CAD build for the part. Positions are in the model's coordinates, mm. Face numbers are marked on the shaded views. A direction names the side the tool comes from. Coordinates: 2 decimals unless noted, no trailing zeros. Loops run counter-clockwise (first coordinate to the right, second up) from the corner with the lowest first, then second, coordinate; pieces in that order, holes last. Notation, with made-up numbers: (62, 0.5) -> (117, 0.5) arc R14 cw to (117, 7.5) -> close; hole circle Ø11 at (-31.5, -29). An arc over 180 degrees is marked (long way). Return JSON: item names as keys, results as strings. Group by question number.
(1) Flat gauge pins, fed straight in: pin 1 Ø4 at (x, y) = (-44, 44) entering from -Z; pin 2 Ø5 at (x, z) = (10, 10) entering from -Y; pin 3 Ø4.5 at (x, z) = (-9, 9) entering from -Y; pin 4 Ø16 at (x, z) = (63.5, 14.5) entering from -Y. Where does each tip first touch, or does it go through?
(2) Saw through at A-A on y = 12. Write the cut outline in (x, z), then the cut area to 3 significant figures.
(3) Saw through at D-D on x = 70. Write the cut outline in (y, z), then the cut area to 3 significant figures.
(4) Saw through at C-C on z = 24. Write the cut outline in (x, y).
(5) Tool access for the marked faces 1, 2, 3 and 4: list every direction of +Z, -Z, +X, -X, +Y, -Y with a clear straight run to the whole face (end or side of a thin tool).
(6) Probe L1, parallel to Z at x = 10, y = -51.2; L2, parallel to Y at x = 0, z = 23.5; L3, parallel to X at y = 22.5, z = 14. List the from-to ranges inside material, lowest first.
(7) Mould opens along Y. For the marked faces 5, 6 and 7 say: pulls with the +Y half, pulls with the -Y half, needs draft (parallel to the pull), parting line crosses it, or undercut.
(8) Saw through at B-B on x = -24. Write the cut outline in (y, z), then the cut area to 3 significant figures.
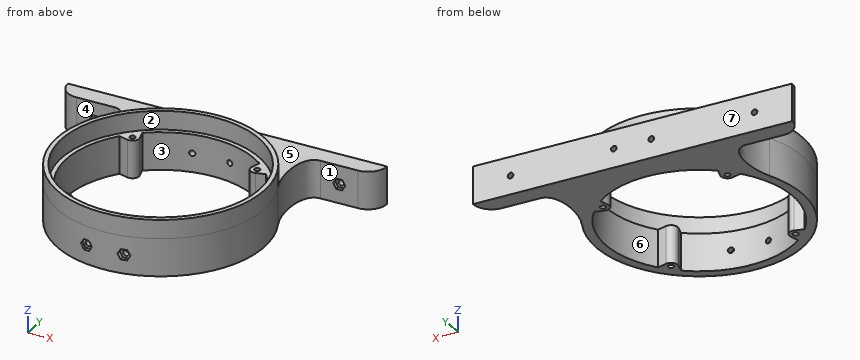
```python
from build123d import *

# Parameters (mm, degrees)
SKETCH_2_R          = 50
EXTRUDE_1_DEPTH     = 20
SKETCH_3_R          = 1.5
CUT_EXTRUDE_1_DEPTH = 149.408220948
SKETCH_4_R          = 1.5
EXTRUDE_2_DEPTH     = 20
CUT_EXTRUDE_START   = -52
CUT_EXTRUDE_4_DEPTH = 57.857705442
CUT_EXTRUDE_5_DEPTH = 2
SKETCH_9_R          = 55
SKETCH_9_R_2        = 50
EXTRUDE_3_DEPTH     = 10
CUT_EXTRUDE_START_2 = -10
SKETCH_10_R         = 52.5
SKETCH_10_R_2       = 50
CUT_EXTRUDE_6_DEPTH = 10


with BuildPart() as part:
    # 草图2 → 凸台-拉伸1 (new body)
    with BuildSketch(Plane.XY):
        with BuildLine():
            Line((-75, 55), (-55, 55))
            add(Edge.make_bspline(
                [(-50, 22.912878475), (-45, 33.823772987), (-45, 55), (-55, 55)],
                knots=[0, 0, 0, 0, 1, 1, 1, 1], degree=3))
            ThreePointArc((-50, 22.912878475), (0, -55), (50, 22.912878475))
            add(Edge.make_bspline(
                [(50, 22.912878475), (45, 33.823772987), (45, 55), (55, 55)],
                knots=[0, 0, 0, 0, 1, 1, 1, 1], degree=3))
            Line((55, 55), (75, 55))
            ThreePointArc((75, 55), (82.071067812, 57.928932188), (85, 65))
            Line((85, 65), (-85, 65))
            ThreePointArc((-85, 65), (-82.071067812, 57.928932188), (-75, 55))
        make_face()
        Circle(SKETCH_2_R, mode=Mode.SUBTRACT)
    extrude(amount=EXTRUDE_1_DEPTH)

    # 草图3 → 切除-拉伸1 (cut, through all)
    with BuildSketch(Plane(origin=(0, 65, 0), x_dir=(1, 0, 0), z_dir=(0, 1, 0))):
        with Locations(Location((-65, -10, 0), (0, 0, 180))):
            Circle(SKETCH_3_R)
        with Locations(Location((-10, -10, 0), (0, 0, 180))):
            Circle(SKETCH_3_R)
        with Locations(Location((10, -10, 0), (0, 0, 180))):
            Circle(SKETCH_3_R)
        with Locations(Location((65, -10, 0), (0, 0, 270))):
            Circle(SKETCH_3_R)
    extrude(amount=-CUT_EXTRUDE_1_DEPTH, mode=Mode.SUBTRACT)

    # 草图4 → 凸台-拉伸2 (add, through all)
    # profile 1 of 4: a face of its own
    with BuildSketch(Plane.XY):
        with BuildLine():
            Line((-31.179095181, 39.087901245), (-29.853278324, 34.139885374))
            ThreePointArc((-29.853278324, 34.139885374), (-30.759144982, 30.759144982), (-34.139885374, 29.853278324))
            Line((-34.139885374, 29.853278324), (-39.087901245, 31.179095181))
            ThreePointArc((-39.087901245, 31.179095181), (-35.355339059, 35.355339059), (-31.179095181, 39.087901245))
        make_face()
        with Locations((-33.234018716, 33.234018716)):
            Circle(SKETCH_4_R, mode=Mode.SUBTRACT)
    # profile 2 of 4: a face of its own
    with BuildSketch(Plane.XY):
        with BuildLine():
            Line((31.179095181, 39.087901245), (29.853278324, 34.139885374))
            ThreePointArc((29.853278324, 34.139885374), (30.759144982, 30.759144982), (34.139885374, 29.853278324))
            Line((34.139885374, 29.853278324), (39.087901245, 31.179095181))
            ThreePointArc((39.087901245, 31.179095181), (35.355339059, 35.355339059), (31.179095181, 39.087901245))
        make_face()
        with Locations((33.234018716, 33.234018716)):
            Circle(SKETCH_4_R, mode=Mode.SUBTRACT)
    # profile 3 of 4: a face of its own
    with BuildSketch(Plane.XY):
        with BuildLine():
            Line((39.087901245, -31.179095181), (34.139885374, -29.853278324))
            ThreePointArc((34.139885374, -29.853278324), (30.759144982, -30.759144982), (29.853278324, -34.139885374))
            Line((29.853278324, -34.139885374), (31.179095181, -39.087901245))
            ThreePointArc((31.179095181, -39.087901245), (35.355339059, -35.355339059), (39.087901245, -31.179095181))
        make_face()
        with Locations((33.234018716, -33.234018716)):
            Circle(SKETCH_4_R, mode=Mode.SUBTRACT)
    # profile 4 of 4: a face of its own
    with BuildSketch(Plane.XY):
        with BuildLine():
            Line((-31.179095181, -39.087901245), (-29.853278324, -34.139885374))
            ThreePointArc((-29.853278324, -34.139885374), (-30.759144982, -30.759144982), (-34.139885374, -29.853278324))
            Line((-34.139885374, -29.853278324), (-39.087901245, -31.179095181))
            ThreePointArc((-39.087901245, -31.179095181), (-35.355339059, -35.355339059), (-31.179095181, -39.087901245))
        make_face()
        with Locations((-33.234018716, -33.234018716)):
            Circle(SKETCH_4_R, mode=Mode.SUBTRACT)
    extrude(amount=EXTRUDE_2_DEPTH)

    # 草图6 → 切除-拉伸4 (cut, through all)
    with BuildSketch(Plane(origin=(0, 0, 0), x_dir=(1, 0, 0), z_dir=(0, 1, 0)).offset(CUT_EXTRUDE_START)):
        Polygon((-8.41228676, -7.25), (-11.58771324, -7.25), (-13.175426481, -10), (-11.58771324, -12.75), (-8.41228676, -12.75), (-6.824573519, -10), align=None)
        Polygon((6.824573519, -10), (8.41228676, -7.25), (11.58771324, -7.25), (13.175426481, -10), (11.58771324, -12.75), (8.41228676, -12.75), align=None)
    extrude(amount=-CUT_EXTRUDE_4_DEPTH, mode=Mode.SUBTRACT)

    # 草图7 → 切除-拉伸5 (cut)
    with BuildSketch(Plane.XZ.offset(-55)):
        Polygon((-63.41228676, 12.75), (-66.58771324, 12.75), (-68.175426481, 10), (-66.58771324, 7.25), (-63.41228676, 7.25), (-61.824573519, 10), align=None)
        Polygon((61.824573519, 10), (63.41228676, 12.75), (66.58771324, 12.75), (68.175426481, 10), (66.58771324, 7.25), (63.41228676, 7.25), align=None)
    extrude(amount=-CUT_EXTRUDE_5_DEPTH, mode=Mode.SUBTRACT)

    # 草图9 → 凸台-拉伸3 (add)
    with BuildSketch(Plane.XY.offset(20)):
        with Locations(Location((0, 0, 0), (0, 0, 155.380022671))):
            Circle(SKETCH_9_R)
        with Locations(Location((0, 0, 0), (0, 0, 218.578178478))):
            Circle(SKETCH_9_R_2, mode=Mode.SUBTRACT)
    extrude(amount=EXTRUDE_3_DEPTH)

    # 草图10 → 切除-拉伸6 (cut)
    with BuildSketch(Plane.XY.offset(30).offset(CUT_EXTRUDE_START_2)):
        Circle(SKETCH_10_R)
        Circle(SKETCH_10_R_2, mode=Mode.SUBTRACT)
    extrude(amount=CUT_EXTRUDE_6_DEPTH, mode=Mode.SUBTRACT)


solid = part.part
```
Geometry results:
{
 "1": {"pin 1": "z = 0", "pin 2": "y = -52", "pin 3": "y = -54.58", "pin 4": "y = 55"},
 "2": {"outline": "(-53.67, 0) -> (-48.54, 0) -> (-48.54, 20) -> (-51.11, 20) -> (-51.11, 30) -> (-53.67, 30) -> close; (48.54, 0) -> (53.67, 0) -> (53.67, 30) -> (51.11, 30) -> (51.11, 20) -> (48.54, 20) -> close", "area": "257 mm²"},
 "3": {"outline": "(55, 0) -> (65, 0) -> (65, 20) -> (55, 20) -> close", "area": "200 mm²"},
 "4": {"outline": "circle Ø110 at (0, 0); hole circle Ø105 at (0, 0)"},
 "5": {"face 1": "+Z, -Z, +X, -Y", "face 2": "+Z", "face 3": "+Z, -Z", "face 4": "+Z, -Z, -X, -Y"},
 "6": {"L1": "0 to 8.5, 11.5 to 20", "L2": "-55 to -52.5, 52.5 to 55", "L3": "-50.19 to -44.65, 44.65 to 50.19"},
 "7": {"face 5": "needs draft", "face 6": "undercut", "face 7": "pulls with the +Y half"},
 "8": {"outline": "(-49.49, 0) -> (-43.86, 0) -> (-43.86, 20) -> (-46.69, 20) -> (-46.69, 30) -> (-49.49, 30) -> close; (43.86, 0) -> (65, 0) -> (65, 20) -> (49.49, 20) -> (49.49, 30) -> (46.69, 30) -> (46.69, 20) -> (43.86, 20) -> close", "area": "591 mm²"}
}
